Can you work these out from the model? Positions are in its coordinate system, mm. A direction names the side the tool comes from. Give positions to 0.01 mm unless a question says otherwise; leave off trailing zeros. Loops run counter-clockwise (first coordinate to the right, second up) from the corner with the lowest first, then second, coordinate; pieces in that order, holes last.
from build123d import *

# Parameters (mm, degrees)
F1_DEPTH = 25.4


with BuildPart() as f1:
    # F0 (on Top) → F1 (new body)
    with BuildSketch(Plane.XY):
        with BuildLine():
            Line((-30.48, 13.97), (-30.48, 0))
            Line((-30.48, 0), (-11.4207109466, 0))
            Line((-11.4207109466, 0), (-11.4207109466, 12.3724368588))
            Line((-11.4207109466, 12.3724368588), (-17.5587640429, 19.0219943798))
            ThreePointArc((-17.5587640429, 19.0219943798), (-23.5431241565, 15.277896023), (-30.48, 13.97))
        make_face()
        Polygon((-11.4207109466, 12.3724368588), (-11.4207109466, 0), (0, 0), align=None)
        with BuildLine():
            ThreePointArc((-17.5587640429, -19.0219943798), (-23.5431241565, -15.277896023), (-30.48, -13.97))
            Line((-30.48, -13.97), (-30.48, -33.02))
            Line((-30.48, -33.02), (-17.5587640429, -19.0219943798))
        make_face()
        with BuildLine():
            Line((-30.48, -33.02), (-30.48, -13.97))
            ThreePointArc((-30.48, -13.97), (-43.9503841816, -46.4903841816), (-11.43, -33.02))
            Line((-11.43, -33.02), (-30.48, -33.02))
        make_face()
        with BuildLine():
            ThreePointArc((-49.53, 33.02), (-43.9503841816, 19.5496158184), (-30.48, 13.97))
            Line((-30.48, 13.97), (-30.48, 33.02))
            Line((-30.48, 33.02), (-49.53, 33.02))
        make_face()
        with BuildLine():
            Line((-30.48, 33.02), (-30.48, 13.97))
            ThreePointArc((-30.48, 13.97), (-23.5431241565, 15.277896023), (-17.5587640429, 19.0219943798))
            Line((-17.5587640429, 19.0219943798), (-30.48, 33.02))
        make_face()
        Polygon((11.4207109466, 12.3724368588), (0, 0), (11.4207109466, 0), align=None)
        Polygon((-11.4207109466, 12.3724368588), (0, 0), (11.4207109466, 12.3724368588), align=None)
        Polygon((11.4207109466, 0), (0, 0), (11.4207109466, -12.3724368588), align=None)
        with BuildLine():
            Line((-17.5587640429, 19.0219943798), (-11.4207109466, 12.3724368588))
            Line((-11.4207109466, 12.3724368588), (11.4207109466, 12.3724368588))
            Line((11.4207109466, 12.3724368588), (17.5587640429, 19.0219943798))
            ThreePointArc((17.5587640429, 19.0219943798), (13.0293260161, 25.3795499145), (11.43, 33.02))
            Line((11.43, 33.02), (-11.43, 33.02))
            ThreePointArc((-11.43, 33.02), (-13.0293260161, 25.3795499145), (-17.5587640429, 19.0219943798))
        make_face()
        with BuildLine():
            Line((11.4207109466, -12.3724368588), (-11.4207109466, -12.3724368588))
            Line((-11.4207109466, -12.3724368588), (-17.5587640429, -19.0219943798))
            ThreePointArc((-17.5587640429, -19.0219943798), (-13.0293260161, -25.3795499145), (-11.43, -33.02))
            Line((-11.43, -33.02), (11.43, -33.02))
            ThreePointArc((11.43, -33.02), (13.0293260161, -25.3795499145), (17.5587640429, -19.0219943798))
            Line((17.5587640429, -19.0219943798), (11.4207109466, -12.3724368588))
        make_face()
        with BuildLine():
            Line((-17.5587640429, -19.0219943798), (-30.48, -33.02))
            Line((-30.48, -33.02), (-11.43, -33.02))
            ThreePointArc((-11.43, -33.02), (-13.0293260161, -25.3795499145), (-17.5587640429, -19.0219943798))
        make_face()
        with BuildLine():
            Line((-49.53, 33.02), (-30.48, 33.02))
            Line((-30.48, 33.02), (-11.43, 33.02))
            ThreePointArc((-11.43, 33.02), (-30.48, 52.07), (-49.53, 33.02))
        make_face()
        with BuildLine():
            Line((-11.43, 33.02), (-30.48, 33.02))
            Line((-30.48, 33.02), (-17.5587640429, 19.0219943798))
            ThreePointArc((-17.5587640429, 19.0219943798), (-13.0293260161, 25.3795499145), (-11.43, 33.02))
        make_face()
        with BuildLine():
            Line((11.4207109466, 12.3724368588), (11.4207109466, 0))
            Line((11.4207109466, 0), (30.48, 0))
            Line((30.48, 0), (30.48, 13.97))
            ThreePointArc((30.48, 13.97), (23.5431241565, 15.277896023), (17.5587640429, 19.0219943798))
            Line((17.5587640429, 19.0219943798), (11.4207109466, 12.3724368588))
        make_face()
        with BuildLine():
            Line((30.48, 0), (11.4207109466, 0))
            Line((11.4207109466, 0), (11.4207109466, -12.3724368588))
            Line((11.4207109466, -12.3724368588), (17.5587640429, -19.0219943798))
            ThreePointArc((17.5587640429, -19.0219943798), (23.5431241565, -15.277896023), (30.48, -13.97))
            Line((30.48, -13.97), (30.48, 0))
        make_face()
        with BuildLine():
            ThreePointArc((17.5587640429, -19.0219943798), (13.0293260161, -25.3795499145), (11.43, -33.02))
            Line((11.43, -33.02), (30.48, -33.02))
            Line((30.48, -33.02), (17.5587640429, -19.0219943798))
        make_face()
        with BuildLine():
            Line((30.48, -33.02), (11.43, -33.02))
            ThreePointArc((11.43, -33.02), (30.48, -52.07), (49.53, -33.02))
            ThreePointArc((49.53, -33.02), (43.9503841816, -19.5496158184), (30.48, -13.97))
            Line((30.48, -13.97), (30.48, -33.02))
        make_face()
        with BuildLine():
            ThreePointArc((11.43, 33.02), (13.0293260161, 25.3795499145), (17.5587640429, 19.0219943798))
            Line((17.5587640429, 19.0219943798), (30.48, 33.02))
            Line((30.48, 33.02), (11.43, 33.02))
        make_face()
        with BuildLine():
            Line((30.48, 33.02), (17.5587640429, 19.0219943798))
            ThreePointArc((17.5587640429, 19.0219943798), (23.5431241565, 15.277896023), (30.48, 13.97))
            Line((30.48, 13.97), (30.48, 33.02))
        make_face()
        with BuildLine():
            ThreePointArc((30.48, -13.97), (23.5431241565, -15.277896023), (17.5587640429, -19.0219943798))
            Line((17.5587640429, -19.0219943798), (30.48, -33.02))
            Line((30.48, -33.02), (30.48, -13.97))
        make_face()
        with BuildLine():
            ThreePointArc((49.53, 33.02), (30.48, 52.07), (11.43, 33.02))
            Line((11.43, 33.02), (30.48, 33.02))
            Line((30.48, 33.02), (49.53, 33.02))
        make_face()
        with BuildLine():
            Line((30.48, 33.02), (30.48, 13.97))
            ThreePointArc((30.48, 13.97), (43.9503841816, 19.5496158184), (49.53, 33.02))
            Line((49.53, 33.02), (30.48, 33.02))
        make_face()
    extrude(amount=F1_DEPTH)


solid = f1.part
(1) Which directions (+Z, -Z, +X, -X, +Y, -Y) give clear straight access to the entire face, cutting with the end or side of a thin tool? Please do faces 4 (the flat face through (0, -33.02, 13)), 5 (the flat face through (0, -12.372, 13)), 6 (the flat face through (-14.447, -15.651, 12.522)).
Returned:
face 4: +Z, -Z, -Y
face 5: +Z, -Z, -X
face 6: +Z, -Z
(2) Thinking about a two-plate mould opening in Y: for faces 1 (the flat face through (0, 33.02, 13)), 2 (the flat face through (-1, 1, 25.4)), 3 (the flat face through (30.48, 0, 13)), which applies, pulls with the +Y half, pulls with the -Y half, needs draft (parallel to the pull), parting line crosses it, or undercut?
Returned:
face 1: pulls with the +Y half
face 2: needs draft
face 3: undercut
(3) Suppose I cut it at B-B on z = 7.75. List the corners of the cut face in (x, y) for me, plus the area to 3 significant figures.
Returned:
outline: (-30.48, 0) - (0, 0) - (11.42, -12.37) - (-11.42, -12.37) - (-17.56, -19.02) arc R19.05 ccw (long way) to (-11.43, -33.02) - (11.43, -33.02) arc R19.05 ccw (long way) to (30.48, -13.97) - (30.48, 13.97) arc R19.05 ccw (long way) to (11.43, 33.02) - (-11.43, 33.02) arc R19.05 ccw (long way) to (-30.48, 13.97) - close
area: 6,940 mm2
(4) Will these pins go through, and if not, where does the flat tip stop? P1, Ø4, axis at y = 5, z = 11, coming from the -X side; P2, Ø12.5, axis at y = -6.5, z = 9, coming from the +X side; P3, Ø6, axis at x = -22.5, z = 13.5, coming from the +Y side.
Returned:
P1: stops at x = -30.48
P2: stops at x = 30.48
P3: stops at y = 51.41
(5) Suppose I cut it at C-C on x = -23. List the corners of the cut face in (y, z) for me, plus the area to 3 significant figures.
Returned:
outline: (-50.54, 0) - (-15.5, 0) - (-15.5, 25.4) - (-50.54, 25.4) - close; (0, 0) - (50.54, 0) - (50.54, 25.4) - (0, 25.4) - close
area: 2,170 mm2
(6) Suppose I cut it at D-D on y = 21. List the corners of the cut face in (x, z) for me, plus the area to 3 significant figures.
Returned:
outline: (-45.26, 0) - (45.26, 0) - (45.26, 25.4) - (-45.26, 25.4) - close
area: 2,300 mm2
(7) Please list where these lines run through material, in increasing order: probe 1 along Y at (x, z) = (-10.5, 17.5); probe 2 along X at (y, z) = (0.5, 6.5); probe 3 along Y at (x, z) = (31.5, 11).
Returned:
probe 1: y = -33.02 to -12.37, 0 to 33.02
probe 2: x = -30.48 to 30.48
probe 3: y = -52.04 to -14, 14 to 52.04
(8) Suppose I cut it at A-A on y = -42.5. List the corners of the cut face in (x, z) for me.
Returned:
outline: (-47, 0) - (-13.96, 0) - (-13.96, 25.4) - (-47, 25.4) - close; (13.96, 0) - (47, 0) - (47, 25.4) - (13.96, 25.4) - close
